Job drawing, mm, ordinate dimensions from the low corner. One solid piece. Coordinates: 2 decimals unless noted, no trailing zeros. Order: outer loops, then holes, each group sorted by start corner. A loop starts at its lowest first (then second) coordinate and runs counter-clockwise, first axis right, second up. Notation, with made-up numbers: (-20, -27) -> (34, -27) arc R26 ccw to (34, -5) -> close; hole circle Ø8 at (57, 48.25). An arc over 180 degrees is marked (long way). Use CSV: the item, a comma, the result in double quotes. Start each with the question number.
(1) Probe L1, parallel to X at y = 94.57, z = 1.1; L2, parallel to X at y = 120.65, z = 1.25 (1 decimal); L3, parallel to Y at x = 62.5, z = 0.7. List the from-to ranges inside material, lowest first.
(2) Cut at A-A on y = 25.4. Write the cut outline in (x, z) (1 decimal), plus the area to 3 significant figures.
(3) Pull direction Z, two halves, no side cores. Call the marked faces 1 and 2: pulls with the +Z half, pulls with the -Z half, needs draft (parallel to the pull), parting line crosses it, or undercut.
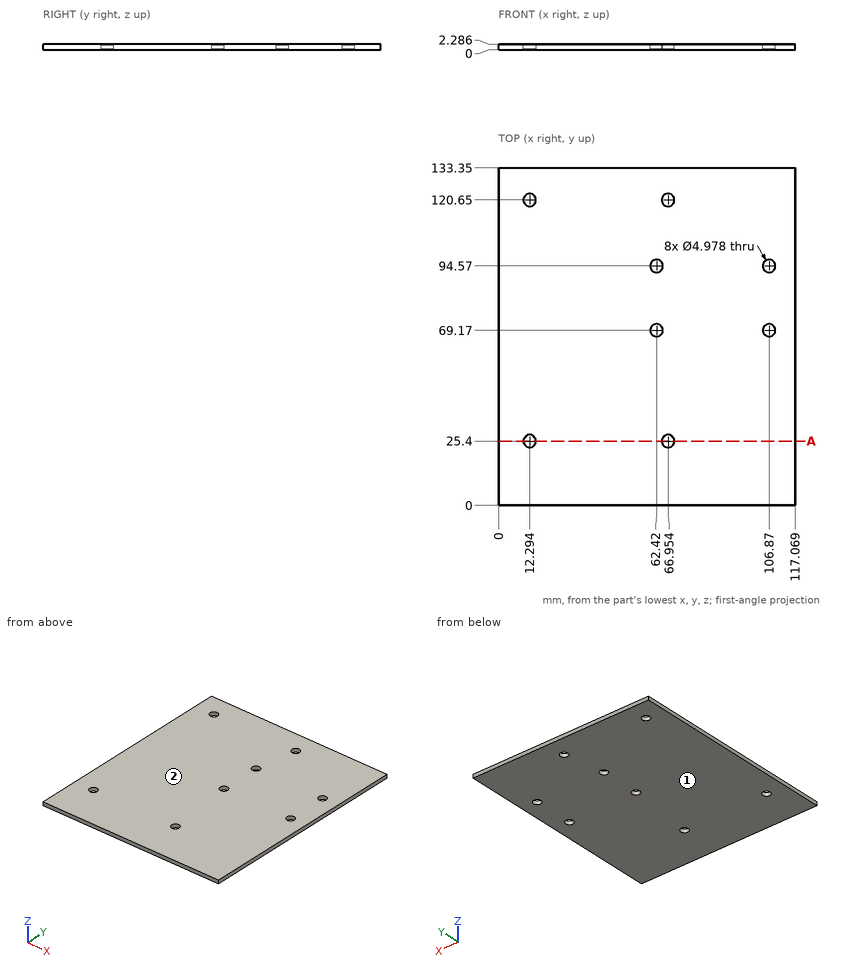
Outcome:
1,L1,"0 to 59.93, 64.91 to 104.38, 109.36 to 117.07"
1,L2,"0 to 9.8, 14.8 to 64.5, 69.4 to 117.1"
1,L3,"0 to 66.68, 71.66 to 92.08, 97.06 to 133.35"
2,outline,"(0, 0) -> (9.8, 0) -> (9.8, 2.3) -> (0, 2.3) -> close; (14.8, 0) -> (64.5, 0) -> (64.5, 2.3) -> (14.8, 2.3) -> close; (69.4, 0) -> (117.1, 0) -> (117.1, 2.3) -> (69.4, 2.3) -> close"
2,area,"245 mm2"
3,face 1,"pulls with the -Z half"
3,face 2,"pulls with the +Z half"
